Geometry: see drawing. Coordinates: mm, zero at the bounding-box minimum. A direction names the side the tool comes from. Round coordinates to 2 decimals unless told otherwise and drop trailing zeros. Order: outer loops, then holes, each group sorted by start corner. A loop starts at its lowest first (then second) coordinate and runs counter-clockwise, first axis right, second up. Notation, with made-up numbers: (89, 33.5) -> (142, 33.5) arc R27 ccw to (142, 54.5) -> close; hole circle Ø3 at (66, 83). An arc over 180 degrees is marked (long way). One line per item, written item: value. Start each with the question number.
1) Ray query, L1, parallel to Z at x = 15, y = 1.2; L2, parallel to X at y = 2, z = 20; L3, parallel to Y at x = 24.25, z = 8.5. Return the intervals inside material, ascending.
2) Section C-C (x = 14.25). Return the cut outline in (y, z).
3) Reachability of the marked faces 1 and 2 from +Z, -Z, +X, -X, +Y, -Y: full face, straight path, thin tool, end or side. Return the list, or none.
4) Pin query (flat end, axial travel): P1, Ø6, axis at x = 20.5, y = 15.5, coming from the -Z side; P2, Ø2, axis at x = 13.5, y = 12, coming from the +Z side; P3, Ø5, axis at x = 15, z = 20, coming from the +Y side; P4, Ø8, axis at x = 9, z = 34, coming from the +Y side. Return the tip coordinate at first contact, or that it passes through.
5) Mould query, pull axis X, two halves, no side actions, for the marked faces 3, 4, 5 and 6. Classes: pulls with the +X half, pulls with the -X half, needs draft (parallel to the pull), parting line crosses it, or undercut.
6) Section D-D (z = 4). Return the cut outline in (x, y).
7) Section A-A (z = 20). Return the cut outline in (x, y), and give its area (3 significant figures).
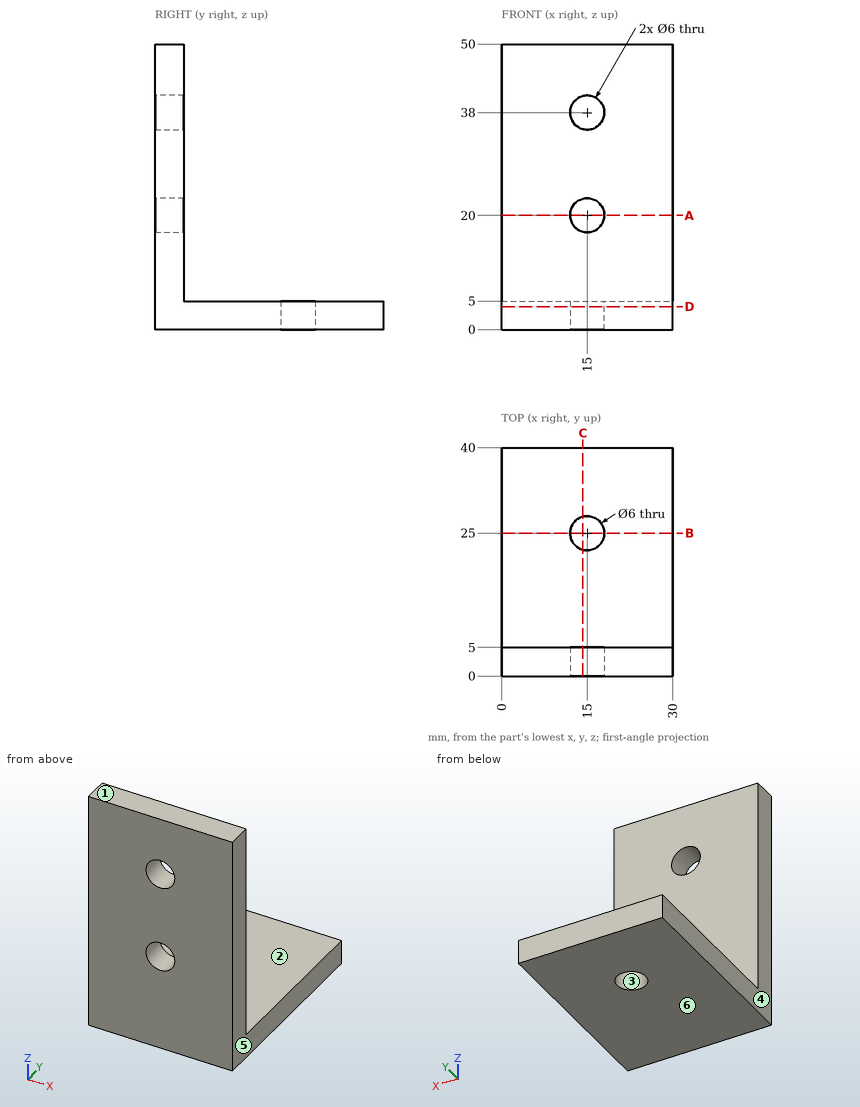
Findings:
1. L1: 0 to 17, 23 to 35, 41 to 50
1. L2: 0 to 12, 18 to 30
1. L3: 0 to 5
2. outline: (0, 0) -> (22.1, 0) -> (22.1, 5) -> (5, 5) -> (5, 17.1) -> (0, 17.1) -> close; (0, 22.9) -> (5, 22.9) -> (5, 35.1) -> (0, 35.1) -> close; (0, 40.9) -> (5, 40.9) -> (5, 50) -> (0, 50) -> close; (27.9, 0) -> (40, 0) -> (40, 5) -> (27.9, 5) -> close
3. face 1: +Z, +X, -X, +Y, -Y
3. face 2: +Z, +X, -X, +Y
4. P1: z = 0
4. P2: z = 5
4. P3: through
4. P4: y = 5
5. face 3: undercut
5. face 4: pulls with the -X half
5. face 5: pulls with the +X half
5. face 6: needs draft
6. outline: (0, 0) -> (30, 0) -> (30, 40) -> (0, 40) -> close; hole circle Ø6 at (15, 25)
7. outline: (0, 0) -> (12, 0) -> (12, 5) -> (0, 5) -> close; (18, 0) -> (30, 0) -> (30, 5) -> (18, 5) -> close
7. area: 120 mm2
